Here's how the part is built. I have some questions about the finished solid (model axes, mm). A direction names the side the tool comes from. Give positions to 0.01 mm unless a question says otherwise; leave off trailing zeros. Write each loop counter-clockwise with the first axis right and the second up, starting at its lowest first coordinate (ties: lowest second). Pieces come first, ordered by that corner, then holes. Notation, with made-up numbers: (31.25, 57) -> (37.25, 57) arc R17 cw to (37.25, 64) -> close; hole circle Ø8 at (-30, -22.5). An arc over 180 degrees is marked (long way). Answer as CSV lines item,"result". Start each with the question number.
from build123d import *

# Parameters (mm, degrees)
SKETCH_2_R          = 1.5
SKETCH_2_R_2        = 2
EXTRUDE_1_DEPTH     = 3
CUT_EXTRUDE_1_DEPTH = 66.833122363


with BuildPart() as part:
    # 草图2 → 凸台-拉伸1 (new body)
    with BuildSketch(Plane.XY):
        with BuildLine():
            Line((-9.965217286, 0.833333333), (-4.982608643, 60.416666667))
            ThreePointArc((-4.982608643, 60.416666667), (0, 65), (4.982608643, 60.416666667))
            Line((4.982608643, 60.416666667), (9.965217286, 0.833333333))
            ThreePointArc((9.965217286, 0.833333333), (0, -10), (-9.965217286, 0.833333333))
        make_face()
        Circle(SKETCH_2_R, mode=Mode.SUBTRACT)
        with Locations((0, 7)):
            Circle(SKETCH_2_R, mode=Mode.SUBTRACT)
        with Locations((7, 0)):
            Circle(SKETCH_2_R, mode=Mode.SUBTRACT)
        with Locations((0, -7)):
            Circle(SKETCH_2_R, mode=Mode.SUBTRACT)
        with Locations((-7, 0)):
            Circle(SKETCH_2_R, mode=Mode.SUBTRACT)
        with Locations((0, 60)):
            Circle(SKETCH_2_R_2, mode=Mode.SUBTRACT)
    extrude(amount=EXTRUDE_1_DEPTH)

    # 草图3 → 切除-拉伸1 (cut, through all)
    with BuildSketch(Plane.XY.offset(3)):
        with BuildLine():
            Line((2.676400777, 15.994901653), (0.996521729, 36.083333333))
            ThreePointArc((0.996521729, 36.083333333), (0, 37), (-0.996521729, 36.083333333))
            Line((-0.996521729, 36.083333333), (-2.676400777, 15.994901653))
            ThreePointArc((-2.676400777, 15.994901653), (-2.379252162, 15.196811544), (-1.574886608, 14.917095299))
            ThreePointArc((-1.574886608, 14.917095299), (0, 15), (1.574886608, 14.917095299))
            ThreePointArc((1.574886608, 14.917095299), (2.379252162, 15.196811544), (2.676400777, 15.994901653))
        make_face()
    extrude(amount=-CUT_EXTRUDE_1_DEPTH, mode=Mode.SUBTRACT)


solid = part.part
Item 1: If we section it at D-D (y = 53): Please give me the cut outline in (x, z).
Item 2: We'd pull the mould along Y, two halves only. Please class faces 3 (the face through (2, 28, 3)), 4 (the face through (0, 65, 1)), 5 (the face through (-1.5, 0.07, 1.48)): released by +Y, released by -Y, zero draft, split by the parting line, or undercut.
Item 3: If we section it at C-C (x = 7): Please give me the cut outline in (y, z), and give its area (3 significant figures).
Item 4: For faces 1 (the face through (1.85, 25.9, 1.52)), 2 (the face through (-7.51, 30.21, 1.48)), which set-ups out of +Z, -Z, +X, -X, +Y, -Y let a thin tool reach every point of the face, with its end or its side?
Item 5: If we section it at A-A (z = 0.65): Please give me the cut outline in (x, y), and give its area (3 significant figures).
Item 6: If I drill on line 1 (X direction, y = 21, z = 2.8); line 2 (X direction, y = 57.5, z = 0.4); line 3 (Y direction, x = 4.25, z = 2.65), over which ranges is the centre line in solid material (lowest first)? Write a range as [from, to].
Item 7: I'm going to push a flat-ended pin straight in: pin 1 (1 mm diameter, centred on x = -4.5, z = 2.5, fed in from +Y). Where does the tip first touch, or does it pass through?
Item 8: If we section it at B-B (y = 0): Please give me the cut outline in (x, z), and give its area (3 significant figures).
Final values:
1,outline,"(-5.6, 0) -> (5.6, 0) -> (5.6, 3) -> (-5.6, 3) -> close"
2,face 3,"zero draft"
2,face 4,"released by +Y"
2,face 5,"undercut"
3,outline,"(-7.14, 0) -> (-1.5, 0) -> (-1.5, 3) -> (-7.14, 3) -> close; (1.5, 0) -> (36.29, 0) -> (36.29, 3) -> (1.5, 3) -> close"
3,area,"121 mm2"
4,face 1,"+Z, -Z"
4,face 2,"+Z, -Z, -X, +Y"
5,outline,"(-9.97, 0.83) arc R10 ccw (long way) to (9.97, 0.83) -> (4.98, 60.42) arc R5 ccw to (-4.98, 60.42) -> close; hole circle Ø3 at (-7, 0); hole (-2.68, 15.99) arc R1 ccw to (-1.57, 14.92) arc R15 cw to (1.57, 14.92) arc R1 ccw to (2.68, 15.99) -> (1, 36.08) arc R1 ccw to (-1, 36.08) -> close; hole circle Ø4 at (0, 60); hole circle Ø3 at (0, -7); hole circle Ø3 at (0, 0); hole circle Ø3 at (0, 7); hole circle Ø3 at (7, 0)"
5,area,"971 mm2"
6,line 1,"[-8.28, -2.26], [2.26, 8.28]"
6,line 2,"[-5.23, 5.23]"
6,line 3,"[-9.05, 62.63]"
7,pin 1,"y = 63"
8,outline,"(-10, 0) -> (-8.5, 0) -> (-8.5, 3) -> (-10, 3) -> close; (-5.5, 0) -> (-1.5, 0) -> (-1.5, 3) -> (-5.5, 3) -> close; (1.5, 0) -> (5.5, 0) -> (5.5, 3) -> (1.5, 3) -> close; (8.5, 0) -> (10, 0) -> (10, 3) -> (8.5, 3) -> close"
8,area,"33.0 mm2"
